Part model, mm, in its own coordinate system. A direction names the side the tool comes from. Coordinates: 2 decimals unless noted, no trailing zeros. Write each loop counter-clockwise with the first axis right and the second up, starting at its lowest first coordinate (ties: lowest second). Pieces come first, ordered by that corner, then holes. Notation, with made-up numbers: (20.5, -24) -> (65.5, -24) arc R23 ccw to (65.5, 4) -> close; hole circle Ø8 at (52, -27). An arc over 180 degrees is marked (long way). Write item = value, one per line. Start each with the question number.
Q1. Pin check, flat tips, straight feed: P1, Ø1.8, axis at x = 1, z = -1, coming from the +Y side (3 decimals); P2, Ø2, axis at y = 0.5, z = 1, coming from the -X side; P3, Ø2, axis at x = 7.83, z = 2.86, coming from the -Y side. Stop position of each tip, or through.
Q2. Band-saw the part on A-A, the plane z = 0. Give the number of separate pieces and of enclosed holes in the cut face, plus the area to 3 significant figures.
Q3. Pull direction Z, two halves, no side cores. Call faces 3 (the flat face through (2, 0, 0)), 4 (the cylindrical face through (-1.953, 3.202, -6.264)), 5 (the cylindrical face through (-2.6, 3.17, 11.73)): released by +Z, released by -Z, zero draft, split by the parting line, or undercut.
Q4. Probe line 1 (Z direction, x = 0, y = 3.55); line 2 (Z direction, x = 0, y = 2.45); line 3 (Z direction, x = -7.5, y = 3.2). List the from-to ranges inside material, lowest first.
Q5. Band-saw the part on B-B, the plane x = -2.54. List the corners of the cut face in (y, z) (3 decimals).
Q6. Tool access for faces 1 (the cylindrical face through (-0.98, 1.077, 4.414)), 2 (the flat face through (1, 4.445, 3)): list every direction of +Z, -Z, +X, -X, +Y, -Y with a clear straight run to the whole face (end or side of a thin tool).
Q7. Band-saw the part on D-D, the plane y = 1.8. List the corners of the cut face in (x, z) (1 decimal).
from build123d import *

# Parameters (mm, degrees)
SKETCH2_R      = 2.921
EXTRUDE1_DEPTH = 1.27
SKETCH3_R      = 1.5875
EXTRUDE2_DEPTH = 5.445
SKETCH4_R      = 0.635
EXTRUDE3_DEPTH = 5.191
SKETCH5_R      = 0.635
EXTRUDE4_DEPTH = 5.191


with BuildPart() as part:
    # Sketch1 → Revolve1 (revolve)
    with BuildSketch(Plane.XY):
        Polygon((0, 0), (0, 4.445), (3.81, 4.445), (3.81, 4.191), (12.0142, 4.191), (12.0142, 2.1844), (4.5212, 2.1844), (4.5212, 0), align=None)
    revolve(axis=Axis((0, 0, 0), (0, 1, 0)))

    # Sketch2 → Extrude1 (cut)
    with BuildSketch(Plane(origin=(0, 4.445, 0), x_dir=(1, 0, 0), z_dir=(0, 1, 0))):
        Circle(SKETCH2_R)
    extrude(amount=-EXTRUDE1_DEPTH, mode=Mode.SUBTRACT)

    # Sketch3 → Extrude2 (cut, through all)
    with BuildSketch(Plane.XZ):
        Circle(SKETCH3_R)
    extrude(amount=-EXTRUDE2_DEPTH, mode=Mode.SUBTRACT)

    # Sketch4 → Extrude3 (cut, through all)
    with BuildSketch(Plane(origin=(0, 4.191, 0), x_dir=(1, 0, 0), z_dir=(0, 1, 0))):
        with Locations((0, 6.985)):
            Circle(SKETCH4_R)
        with Locations((-7.825828211, 2.8575)):
            Circle(SKETCH4_R)
        with Locations((-8.3312, 0)):
            Circle(SKETCH4_R)
        with Locations((-7.825828211, -2.8575)):
            Circle(SKETCH4_R)
        with Locations((7.825828211, 2.8575)):
            Circle(SKETCH4_R)
        with Locations((8.3312, 0)):
            Circle(SKETCH4_R)
        with Locations((7.825828211, -2.8575)):
            Circle(SKETCH4_R)
        with Locations((2.54, 6.506813736)):
            Circle(SKETCH4_R)
        with Locations((-2.54, 6.506813736)):
            Circle(SKETCH4_R)
        with Locations((2.54, -6.506813736)):
            Circle(SKETCH4_R)
        with Locations((0, -6.985)):
            Circle(SKETCH4_R)
        with Locations((-2.54, -6.506813736)):
            Circle(SKETCH4_R)
    extrude(amount=-EXTRUDE3_DEPTH, mode=Mode.SUBTRACT)

    # Sketch5 → Extrude4 (cut, through all)
    with BuildSketch(Plane(origin=(0, 4.191, 0), x_dir=(1, 0, 0), z_dir=(0, 1, 0))):
        with Locations((0, 9.525)):
            Circle(SKETCH5_R)
        with Locations((3.4925, 8.861606443)):
            Circle(SKETCH5_R)
        with Locations((-3.4925, 8.861606443)):
            Circle(SKETCH5_R)
        with Locations((3.4925, -8.861606443)):
            Circle(SKETCH5_R)
        with Locations((0, -9.525)):
            Circle(SKETCH5_R)
        with Locations((-3.4925, -8.861606443)):
            Circle(SKETCH5_R)
    extrude(amount=-EXTRUDE4_DEPTH, mode=Mode.SUBTRACT)


solid = part.part
Ans:
q1.P1 = 3.175
q1.P2 = -4.52
q1.P3 = 2.18
q2.separate_pieces = 4
q2.enclosed_holes = 0
q2.area = 47.3 mm2
q3.face_3 = zero draft
q3.face_4 = undercut
q3.face_5 = split by the parting line
q4.line_1 = -12.01 to -10.16, -8.89 to -7.62, -6.35 to -2.92, 2.92 to 6.35, 7.62 to 8.89, 10.16 to 12.01
q4.line_2 = -12.01 to -10.16, -8.89 to -7.62, -6.35 to -1.59, 1.59 to 6.35, 7.62 to 8.89, 10.16 to 12.01
q4.line_3 = -9.39 to -3.4, -2.31 to 2.31, 3.4 to 9.39
q5.outline = (0, -3.74) -> (2.184, -3.74) -> (2.184, -5.872) -> (4.191, -5.872) -> (4.191, -2.84) -> (4.445, -2.84) -> (4.445, -1.442) -> (3.175, -1.442) -> (3.175, 1.442) -> (4.445, 1.442) -> (4.445, 2.84) -> (4.191, 2.84) -> (4.191, 5.872) -> (2.184, 5.872) -> (2.184, 3.74) -> (0, 3.74) -> close; (2.184, -11.743) -> (4.191, -11.743) -> (4.191, -7.142) -> (2.184, -7.142) -> close; (2.184, 7.142) -> (4.191, 7.142) -> (4.191, 11.743) -> (2.184, 11.743) -> close
q6.face_1 = -Y
q6.face_2 = +Z, -Z, +X, -X, +Y
q7.outline = circle Ø9 at (0, 0); hole circle Ø3.2 at (0, 0)
